Design review of the part built by this model. Coordinates are the model's own, in mm. A direction names the side the tool comes from. Give positions to 0.01 mm unless a question says otherwise; leave off trailing zeros. Write each loop counter-clockwise with the first axis right and the second up, starting at its lowest first coordinate (ties: lowest second). Pieces come first, ordered by that corner, then holes. Notation, with made-up numbers: M 10,21.25 L 17,21.25 A32 cw 17,55.25 Z; hole C -26,37.5 d3. An arc over 180 degrees is marked long. Use a Markdown table: item, result. Add a question column.
```python
from build123d import *

# Parameters (mm, degrees)
SALIENTE_EXTRUIR1_DEPTH = 10
CROQUIS1_10_R           = 5
CORTAR_EXTRUIR1_DEPTH   = 6


with BuildPart() as part:
    # Croquis1 → Saliente-Extruir1 (new body)
    with BuildSketch(Plane(origin=(0, 0, 0), x_dir=(1, 0, 0), z_dir=(0, 1, 0))):
        with BuildLine():
            Line((-60.914821384, -22.524031449), (-40.914821384, -22.524031449))
            Line((-40.914821384, -22.524031449), (-40.914821384, -34.524031449))
            Line((-40.914821384, -34.524031449), (-12.914821384, -34.524031449))
            Line((-12.914821384, -34.524031449), (-12.914821384, -22.524031449))
            Line((-12.914821384, -22.524031449), (7.085178616, -22.524031449))
            Line((7.085178616, -22.524031449), (7.085178616, -34.524031449))
            Line((7.085178616, -34.524031449), (35.085178616, -34.524031449))
            Line((35.085178616, -34.524031449), (35.085178616, -22.524031449))
            Line((35.085178616, -22.524031449), (55.085178616, -22.524031449))
            Line((55.085178616, -22.524031449), (55.085178616, -34.524031449))
            Line((55.085178616, -34.524031449), (83.085178616, -34.524031449))
            Line((83.085178616, -34.524031449), (83.085178616, -22.524031449))
            Line((83.085178616, -22.524031449), (103.085178616, -22.524031449))
            Line((103.085178616, -22.524031449), (103.085178616, 62.217775428))
            Line((103.085178616, 62.217775428), (71.349410248, 62.217775428))
            ThreePointArc((71.349410248, 62.217775428), (69.870831169, 63.28983211), (69.085178616, 64.938544239))
            Line((69.085178616, 64.938544239), (69.085178616, 94.127666629))
            Line((69.085178616, 94.127666629), (-26.914821384, 94.127666629))
            Line((-26.914821384, 94.127666629), (-26.914821384, 64.848788639))
            ThreePointArc((-26.914821384, 64.848788639), (-27.737578388, 63.243349526), (-29.221681351, 62.217775428))
            Line((-29.221681351, 62.217775428), (-60.914821384, 62.217775428))
            Line((-60.914821384, 62.217775428), (-60.914821384, -22.524031449))
        make_face()
    extrude(amount=SALIENTE_EXTRUIR1_DEPTH)

    # Croquis1_10 → Cortar-Extruir1 (cut)
    with BuildSketch(Plane(origin=(0, 0, 0), x_dir=(1, 0, 0), z_dir=(0, 1, 0))):
        with Locations(Location((0, 35.380497461, 0), (0, 0, 270))):
            Circle(CROQUIS1_10_R)
        with Locations(Location((40, 35.380497461, 0), (0, 0, 270))):
            Circle(CROQUIS1_10_R)
    extrude(amount=CORTAR_EXTRUIR1_DEPTH, mode=Mode.SUBTRACT)


solid = part.part
```
(1) For pin 1 (3 mm diameter, centred on y = 5.5, z = 27, fed in from -X); pin 2 (5 mm diameter, centred on x = -2, z = -35.5, fed in from -Y); pin 3 (3 mm diameter, centred on y = 3, z = 25.5, fed in from +X), all flat-tipped, find the tip position at first contact; note any pin that passes through.
(2) Add section B-B on x = 40. Give the boundary of the cut face in (y, z), then the cut area to 3 significant figures.
(3) The part is to be moulded in two halves that separate along X. For faces 5 (the flat face through (69.085, 5, -79)), 6 (the flat face through (7.085, 5, 28)), 7 (the flat face through (-60.915, 5, -20)), 8 (the flat face through (-3, 5, 22.524)), say which applies: released by +X, released by -X, zero draft, split by the parting line, or undercut.
(4) Add section A-A on y = 2.5. Give the boundary of the cut face in (x, z), then the cut area to 3 significant figures.
(5) Add section C-C on x = 92. Give the boundary of the cut face in (y, z), then the cut area to 3 significant figures.
(6) Machinability: for faces 1 (the cylindrical face through (1.5, 2.96, -30.61)), 2 (the flat face through (-45, 5, -62.218)), 3 (the flat face through (35.085, 5, 29)), 4 (the flat face through (93, 5, 22.524)), which of the approach directions +Z, -Z, +X, -X, +Y, -Y give a long, thin tool a straight path to every point of the face, cutting with its end or side? Answer none if there is none.
(7) Wall thickness on L1, parallel to X at y = 7, z = 24; L2, parallel to X at y = 3.5, z = -34; L3, parallel to X at y = 6, z = -71.5: over which ranges is each line inside the solid? List them lowest first.
From the geometry:
| question | item | result |
|---|---|---|
| 1 | pin 1 | stops at x = -40.91 |
| 1 | pin 2 | stops at y = 6 |
| 1 | pin 3 | stops at x = 83.09 |
| 2 | outline | M 0,-94.13 L 10,-94.13 L 10,22.52 L 0,22.52 L 0,-30.38 L 6,-30.38 L 6,-40.38 L 0,-40.38 Z |
| 2 | area | 1,110 mm^2 |
| 3 | face 5 | released by +X |
| 3 | face 6 | undercut |
| 3 | face 7 | released by -X |
| 3 | face 8 | undercut |
| 4 | outline | M -60.91,-62.22 L -29.22,-62.22 A3.7 cw -26.91,-64.85 L -26.91,-94.13 L 69.09,-94.13 L 69.09,-64.94 A3.7 cw 71.35,-62.22 L 103.09,-62.22 L 103.09,22.52 L 83.09,22.52 L 83.09,34.52 L 55.09,34.52 L 55.09,22.52 L 35.09,22.52 L 35.09,34.52 L 7.09,34.52 L 7.09,22.52 L -12.91,22.52 L -12.91,34.52 L -40.91,34.52 L -40.91,22.52 L -60.91,22.52 Z; hole C 0,-35.38 d10; hole C 40,-35.38 d10 |
| 4 | area | 17,800 mm^2 |
| 5 | outline | M 0,-62.22 L 10,-62.22 L 10,22.52 L 0,22.52 Z |
| 5 | area | 847 mm^2 |
| 6 | face 1 | -Y |
| 6 | face 2 | -Z, -X, +Y, -Y |
| 6 | face 3 | +Z, +Y, -Y |
| 6 | face 4 | +Z, +X, +Y, -Y |
| 7 | L1 | x = -40.91 to -12.91, 7.09 to 35.09, 55.09 to 83.09 |
| 7 | L2 | x = -60.91 to -4.81, 4.81 to 35.19, 44.81 to 103.09 |
| 7 | L3 | x = -26.91 to 69.09 |
